Check sheet for the modelled part. Datum: model origin and axes. Units: mm. A direction names the side the tool comes from. Give positions to 0.01 mm unless a question says otherwise; leave off trailing zeros. Loops run counter-clockwise (first coordinate to the right, second up) from the corner with the lowest first, then second, coordinate; pieces in that order, holes last. Notation, with made-up numbers: (48, 22) - (75, 22) arc R15 cw to (75, 36) - close; hole circle Ø1 at (34, 28.5). An arc over 180 degrees is marked (long way). Use CSV: the item, a comma, the result in double quotes.
from build123d import *

# Parameters (mm, degrees)
F1_DEPTH = 203.2
F2_W     = 6.35
F2_H     = 25.4
F3_DEPTH = 127


with BuildPart() as f1:
    # F0 (on Front) → F1 (new body)
    with BuildSketch(Plane.XZ):
        Polygon((39.0150669992, 120.0144297529), (-169.0698442861, -25.6450007532), (-110.8060720837, -108.8789652674), (73.4977095011, 20.1336752934), (97.2788392016, 36.7804652388), align=None)
        Polygon((73.4977095011, 20.1336752934), (-110.8060720837, -108.8789652674), (-22.2213511689, -108.8789652674), (102.6295956023, -21.4833069637), align=None)
    extrude(amount=F1_DEPTH)

    # F2 (on face) → F3 (cut)
    with BuildSketch(Plane(origin=(58.786096923, 0, 41.1502657574), x_dir=(0, 1, 0), z_dir=(0.8192319342, 0, 0.5734623248))):
        with Locations((-190.5, -51.0540176069)):
            Rectangle(F2_W, F2_H)
        with Locations((-165.1, -51.0540176069)):
            Rectangle(F2_W, F2_H)
        with Locations((-139.7, -51.0540176069)):
            Rectangle(F2_W, F2_H)
        with Locations((-114.3, -51.0540176069)):
            Rectangle(F2_W, F2_H)
        with Locations((-88.9, -51.0540176069)):
            Rectangle(F2_W, F2_H)
        with Locations((-63.5, -51.0540176069)):
            Rectangle(F2_W, F2_H)
        with Locations((-38.1, -51.0540176069)):
            Rectangle(F2_W, F2_H)
        with Locations((-12.7, -51.0540176069)):
            Rectangle(F2_W, F2_H)
    extrude(amount=-F3_DEPTH, mode=Mode.SUBTRACT)


solid = f1.part
1. Sectioned sample at A-A, the plane x = 64.5. State how many separate pieces and enclosed holes the cut face has, and give its area (3 significant figures).
Completed:
separate pieces,"1"
enclosed holes,"8"
area,"25,200 mm²"
2. Release check for a two-part mould opening along Z. For faces 4 (the face through (-63.571, -100.178, 48.204)), 5 (the face through (29.488, -88.944, -26.176)), 6 (the face through (-35, 0, -18)) record: released by +Z, released by -Z, zero draft, split by the parting line, or undercut.
Completed:
face 4,"released by +Z"
face 5,"undercut"
face 6,"zero draft"
3. Sectioned sample at D-D, the plane z = 41. Record the boundary of the cut face in (x, y).
Completed:
outline,"(-73.86, -203.2) - (94.33, -203.2) - (94.33, 0) - (-73.86, 0) - close"
4. Sectioned sample at C-C, the plane x = -128. Record the boundary of the cut face in (y, z).
Completed:
outline,"(-203.2, -84.32) - (0, -84.32) - (0, 3.1) - (-203.2, 3.1) - close"
5. Go/stop test with flat-tipped pins: pin 1 Ø4 at (x, y) = (29, -148.5) entering from +Z; pin 2 Ø2 at (x, y) = (-44.5, -33) entering from +Z; pin 3 Ø1 at (y, z) = (-30.5, -23.5) entering from +X. Record where each tip stops, or that it passes through.
Completed:
pin 1,"stops at z = 114.4"
pin 2,"stops at z = 62.25"
pin 3,"stops at x = 100.46"
6. Scan lines: line 1 along X through (y, z) = (-89, -41); line 2 along X through (y, z) = (-89, -20.5); line 3 along Z through (x, y) = (45.5, -138.5). Record each from-to range of solid material in increasing order.
Completed:
line 1,"x = -158.32 to 8.31, 52.6 to 74.75"
line 2,"x = -161.72 to 37.6, 81.89 to 101.94"
line 3,"z = -61.47 to -45.97, -14.97 to 110.75"
7. Set-up check for faces 1 (the face through (85.22, -100.18, 28.34)), 2 (the face through (39.33, -100.178, -65.793)), 3 (the face through (44.054, -38.144, -46.984)): record each of +Z, -Z, +X, -X, +Y, -Y from which the full face is reachable in a straight line by a thin tool's end or side.
Completed:
face 1,"+X, +Y, -Y"
face 2,"-Z, +X, +Y, -Y"
face 3,"none"
